Read the model definition and answer for the solid it produces. Units are mm, in the model's axes. A direction names the side the tool comes from. Give positions to 0.01 mm unless a question says otherwise; leave off trailing zeros. Order: outer loops, then holes, each group sorted by start corner. A loop starts at its lowest first (then second) coordinate and runs counter-clockwise, first axis right, second up.
```python
from build123d import *

# Parameters (mm, degrees)
SKETCH1_R           = 1.4224
BOSS_EXTRUDE1_DEPTH = 3.175


with BuildPart() as part:
    # Sketch1 → Boss-Extrude1 (new body)
    with BuildSketch(Plane.XY):
        Polygon((6075.440076302, 2666.732382812), (6075.440076302, 2669.907382812), (6023.357376302, 2669.907382812), (6023.357376302, 2666.732382812), (6020.182376302, 2666.732382812), (6020.182376302, 2669.907382812), (5971.279772433, 2669.907382812), (5971.279772433, 2666.732382812), (5968.104772433, 2666.732382812), (5968.104772433, 2669.907382812), (5914.429476302, 2669.907382812), (5914.429476302, 2666.732382812), (5907.622276302, 2666.732382812), (5907.622276302, 2657.537582812), (6082.247276302, 2657.537582812), (6082.247276302, 2666.732382812), align=None)
        with Locations((5995.731074367, 2662.134982812)):
            Circle(SKETCH1_R, mode=Mode.SUBTRACT)
        with Locations((5917.604476302, 2662.134982812)):
            Circle(SKETCH1_R, mode=Mode.SUBTRACT)
        with Locations((6072.265076302, 2662.134982812)):
            Circle(SKETCH1_R, mode=Mode.SUBTRACT)
    extrude(amount=BOSS_EXTRUDE1_DEPTH)


solid = part.part
```
1) A tool of negligible diameter and unlimited length cuts with its end or side. For faces 1 (the face through (5971.28, 2668, 2)), 2 (the face through (5994, 2664, 0)), from which of +Z, -Z, +X, -X, +Y, -Y can it reach the whole face along a straight path? Write none if from no direction.
Final values:
face 1: +Z, -Z, +Y
face 2: -Z, +X, -X, +Y, -Y
2) Consider L1, parallel to X at y = 2662.25, z = 0.5; L2, parallel to X at y = 2668.75, z = 1.95; L3, parallel to X at y = 2663, z = 1.25. Determine where each line is inside the solid, lowest interval first.
Final values:
L1: x = 5907.62 to 5916.19, 5919.02 to 5994.31, 5997.15 to 6070.85, 6073.68 to 6082.25
L2: x = 5914.43 to 5968.1, 5971.28 to 6020.18, 6023.36 to 6075.44
L3: x = 5907.62 to 5916.48, 5918.73 to 5994.6, 5996.86 to 6071.14, 6073.39 to 6082.25
3) Given pin 1 (1 mm diameter, centred on y = 2668, z = 1.5, fed in from -X); pin 2 (1 mm diameter, centred on y = 2668.5, z = 1, fed in from +X); pin 3 (1.6 mm diameter, centred on x = 5910, z = 1.5, fed in from +Y), each flat-ended and moving along its own axis, determine where each tip first touches the part or whether it passes through.
Final values:
pin 1: stops at x = 5914.43
pin 2: stops at x = 6075.44
pin 3: stops at y = 2666.73
4) The part is cut by section A-A on z = 2.2. Determine the outline of the cut face in (x, y), and give its area (3 significant figures).
Final values:
outline: (5907.62, 2657.54) - (6082.25, 2657.54) - (6082.25, 2666.73) - (6075.44, 2666.73) - (6075.44, 2669.91) - (6023.36, 2669.91) - (6023.36, 2666.73) - (6020.18, 2666.73) - (6020.18, 2669.91) - (5971.28, 2669.91) - (5971.28, 2666.73) - (5968.1, 2666.73) - (5968.1, 2669.91) - (5914.43, 2669.91) - (5914.43, 2666.73) - (5907.62, 2666.73) - close; hole circle Ø2.84 at (5917.6, 2662.13); hole circle Ø2.84 at (5995.73, 2662.13); hole circle Ø2.84 at (6072.27, 2662.13)
area: 2,080 mm2
5) For a pull along X with two mould halves and no side action, classify faces 3 (the face through (6075.44, 2668, 2)), 4 (the face through (5914.429, 2668, 2)), 5 (the face through (6022, 2666.732, 2)), 6 (the face through (6023.357, 2668, 2)) as released by +X, released by -X, zero draft, split by the parting line, or undercut.
Final values:
face 3: released by +X
face 4: released by -X
face 5: undercut
face 6: undercut
